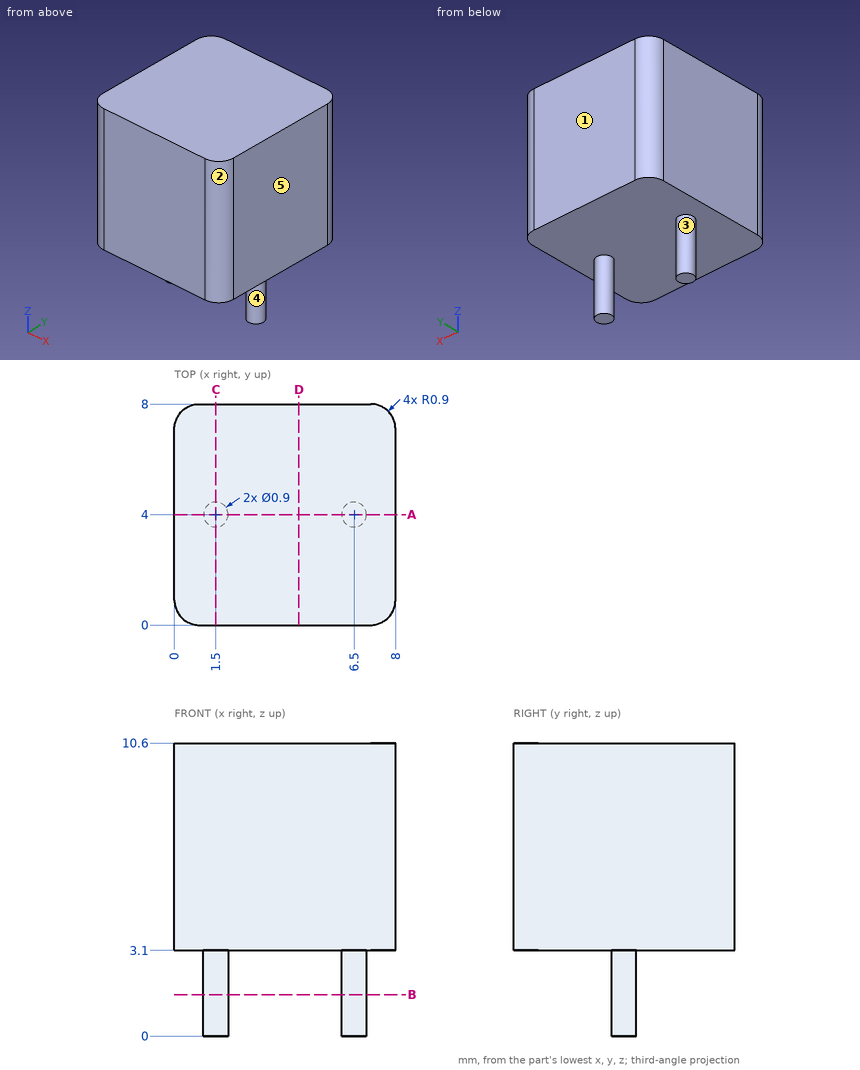
Source: three-view drawing plus pictorial views. Frame: mm from the lowest corner of the part. A direction names the side the tool comes from. Round coordinates to 2 decimals unless told otherwise and drop trailing zeros. Order: outer loops, then holes, each group sorted by start corner. A loop starts at its lowest first (then second) coordinate and runs counter-clockwise, first axis right, second up. Notation, with made-up numbers: (13, -30) -> (56, -30) arc R25 cw to (56, 9) -> close; hole circle Ø5 at (79, -32). An arc over 180 degrees is marked (long way). Use one line per item in the form item = value.
(1) Ray query, probe 1 along Z at (x, y) = (0.5, 1.5); probe 2 along Y at (x, z) = (1.5, 0.75); probe 3 along X at (y, z) = (7.5, 3.5). Return the intervals inside material, ascending. Write a range as [from, to].
Results list:
probe_1 = [3.1, 10.6]
probe_2 = [3.55, 4.45]
probe_3 = [0.09, 7.91]
(2) Draft query along X for the marked faces 1, 2 and 3. Return one class per face: pulls with the +X half, pulls with the -X half, needs draft (parallel to the pull), parting line crosses it, or undercut.
Results list:
face_1 = needs draft
face_2 = pulls with the +X half
face_3 = undercut
(3) Section C-C on x = 1.5. Return loops of the section in (y, z).
Results list:
outline = (0, 3.1) -> (3.55, 3.1) -> (3.55, 0) -> (4.45, 0) -> (4.45, 3.1) -> (8, 3.1) -> (8, 10.6) -> (0, 10.6) -> close
(4) Section D-D on x = 4.5. Return loops of the section in (y, z), and give its area (3 significant figures).
Results list:
outline = (0, 3.1) -> (8, 3.1) -> (8, 10.6) -> (0, 10.6) -> close
area = 60.0 mm^2
(5) Section A-A on y = 4. Return loops of the section in (x, z), and give its area (3 significant figures).
Results list:
outline = (0, 3.1) -> (1.05, 3.1) -> (1.05, 0) -> (1.95, 0) -> (1.95, 3.1) -> (6.05, 3.1) -> (6.05, 0) -> (6.95, 0) -> (6.95, 3.1) -> (8, 3.1) -> (8, 10.6) -> (0, 10.6) -> close
area = 65.6 mm^2
(6) Section B-B on z = 1.5. Return loops of the section in (x, y).
Results list:
outline = circle Ø0.9 at (1.5, 4); circle Ø0.9 at (6.5, 4)
(7) Access query for the marked faces 4 and 5. Directions: +Z, -Z, +X, -X, +Y, -Y. A direction counts if a zero-diameter tool reaches every point of the face in a straight line with its end or side. Return the directions, or none.
Results list:
face_4 = -Z
face_5 = +Z, -Z, +X, +Y, -Y
(8) First-contact query: pin 1 Ø1.5 at (x, y) = (5.5, 3) entering from -Z. Flat tip, straight axial feed; report the tip coordinate or a pass-through.
Results list:
pin_1 = 3.1
